CAD build for the part. Positions are in the model's coordinates, mm. A direction names the side the tool comes from. Coordinates: 2 decimals unless noted, no trailing zeros. Order: outer loops, then holes, each group sorted by start corner. A loop starts at its lowest first (then second) coordinate and runs counter-clockwise, first axis right, second up. Notation, with made-up numbers: M -38.75,32 L -22.75,32 A20 cw -22.75,38 Z; hole C 3,77.25 d9. An arc over 180 degrees is marked long. Write item = value, one per line.
Autodesk Inventor part; units mm, degrees
ref_plane "WorkPlane1" through (0, 0, 0) normal (0, 0, 1) x (1, 0, 0)
ref_plane "Work Plane2" through (0, 0, -1.3) normal (0, 0, 1) x (1, 0, 0)
ref_plane "WorkPlane2" through (0, 0, 1) normal (0, 0, 1) x (1, 0, 0)
ref_plane "WorkPlane1" through (0, 0, 0) normal (0, 0, 1) x (1, 0, 0)
ref_plane "Work Plane2" through (0, 0, -1.3) normal (0, 0, 1) x (1, 0, 0)
ref_plane "WorkPlane2" through (0, 0, 1) normal (0, 0, 1) x (1, 0, 0)
sketch "Szkic1" plane through (0, 0, 0) normal (0, 0, 1) x (1, 0, 0)
  point P0 (0, 0)
sketch "Szkic2" plane through (0, 0, 0) normal (0, 0, 1) x (1, 0, 0)
  line L0 (6.5, -14.9542) -> (5.6095, -12.8096)
  arc A0 (8.8615, -10.0274) -> (5.6095, -12.8096) centre (7.6875, -11.9468) ccw
  line L1 (8.8615, -10.0274) -> (10.3425, -10.9332)
  arc A1 (10.3425, -10.9332) -> (-10.3425, -10.9332) centre (0, 0) ccw
  line L2 (-8.8615, -10.0274) -> (-10.3425, -10.9332)
  arc A2 (-5.6095, -12.8096) -> (-8.8615, -10.0274) centre (-7.6875, -11.9468) ccw
  line L3 (-6.5, -14.9542) -> (-5.6095, -12.8096)
  arc A3 (6.5, -14.9542) -> (-6.5, -14.9542) centre (0, 0.7) ccw
  line L4 (0, 0.7) -> (-6.5, -14.9542) construction
  line L5 (0, 0.7) -> (6.5, -14.9542) construction
  dimension "d2" = 16.95
  dimension "d4" = 0
  dimension "d6" = 15.05
  dimension "d8" = 0.7
  dimension "d10" = 6.5
  dimension "d12" = 6.5
  dimension "d14" = 2.25
  dimension "d16" = 2.25
  dimension "d18" = 14.8
  dimension "d20" = 14.8
  dimension "d22" = 36
  dimension "d24" = 36
extrude "Wyciągnięcie proste1" add sketch "Szkic2" along normal blind 1.3
sketch "Szkic3" plane through (0, 0, 1.3) normal (0, 0, 1) x (1, 0, 0)
  arc A0 (-5.6095, -12.8096) -> (-8.8615, -10.0274) centre (-7.6875, -11.9468) ccw
hole "Otwór1" at (-7.6875, -11.9468, 1.3) direction (0, 0, -1) diameter 2.5 end through all
sketch "Szkic4" plane through (0, 0, 1.3) normal (0, 0, 1) x (1, 0, 0)
  arc A0 (8.8615, -10.0274) -> (5.6095, -12.8096) centre (7.6875, -11.9468) ccw
hole "Otwór2" at (7.6875, -11.9468, 1.3) direction (0, 0, -1) diameter 2.5 end through all
equation "\"d2\" = 0.5 * Diam2"
equation "\"d6\" = 0.5 * msp_dd1"
equation "\"d8\" = -0.5 * msp_dd1 + 0.5 * Diam2 - 0.222222 * ParA"
equation "\"d10\" = 2.6 * Diam5"
equation "\"d12\" = 2.6 * Diam5"
equation "\"d14\" = 0.9 * Diam5"
equation "\"d16\" = 0.9 * Diam5"
equation "\"d18\" = 1.3 * Diam5 + 0.5 * Diam2 - ParA"
equation "\"d20\" = 1.3 * Diam5 + 0.5 * Diam2 - ParA"
equation "\"d25\" = ParS"
equation "\"d29\" = Diam5"
equation "\"d36\" = Diam5"
equation "\"Diam5\" = 2.5"
equation "\"ParA\" = 5.4"
equation "\"ParS\" = 1.3"
equation "\"Diam2\" = 33.9"
equation "\"msp_dd1\" = -b + Diam2 - 0.111111 * ParA"
equation "\"msp_pom\" = 0.5 * Diam2 - b"
equation "\"TEMPLATE\" = 1.2345"
properties part number "ANSI B 27.7M - 3BMI-32" material "Stal, miękka"
(1) Slice it at C-C, the plane z = 0.4. Write the cut outline in (x, y).
Evaluation:
outline = M -10.34,-10.93 A15.05 cw long 10.34,-10.93 L 8.86,-10.03 A2.25 ccw 5.61,-12.81 L 6.5,-14.95 A16.95 ccw long -6.5,-14.95 L -5.61,-12.81 A2.25 ccw -8.86,-10.03 Z; hole C -7.69,-11.95 d2.5; hole C 7.69,-11.95 d2.5
(2) Pin check, flat tip, straight feed: pin 1 Ø10 at (x, y) = (7.5, 3) entering from +Z. Stop position of the tip, or through.
Evaluation:
pin_1 = through
(3) Slice it at D-D, the plane x = 0. Write the cut outline in (y, z).
Evaluation:
outline = M 15.05,0 L 17.65,0 L 17.65,1.3 L 15.05,1.3 Z
(4) Tool access for faces 1 (the face through (6.061, -13.897, 0.641)), 2 (the face through (-4, 15, 0)), 3 (the face through (9.592, -10.474, 0.641)): list every direction of +Z, -Z, +X, -X, +Y, -Y with a clear straight run to the whole face (end or side of a thin tool).
Evaluation:
face_1 = +Z, -Z, -Y
face_2 = -Z, +X, -X, +Y, -Y
face_3 = +Z, -Z
(5) Wall check: line 1 (X direction, y = 0.5, z = 0.5); line 2 (Y direction, x = -8.5, z = 0.3); line 3 (X direction, y = -12.5, z = 0.85). Give the ranges that are in metal, low to high. Write a range as from..to.
Evaluation:
line_1 = -16.95..-15.04, 15.04..16.95
line_2 = -13.96..-12.9, -11..-9.85, 12.42..15.36
line_3 = -10.63..-8.81, -6.57..-5.51, 5.51..6.57, 8.81..10.63
(6) Slice it at A-A, the plane y = 12. Write the cut outline in (x, z), then the cut area to 3 significant figures.
Evaluation:
outline = M -12.63,0 L -9.08,0 L -9.08,1.3 L -12.63,1.3 Z; M 9.08,0 L 12.63,0 L 12.63,1.3 L 9.08,1.3 Z
area = 9.23 mm²
(7) Slice it at B-B, the plane x = -11.5. Write the cut outline in (y, z).
Evaluation:
outline = M -11.75,0 L -9.71,0 L -9.71,1.3 L -11.75,1.3 Z; M 9.71,0 L 13.15,0 L 13.15,1.3 L 9.71,1.3 Z
(8) Pull direction X, two halves, no side cores. Call faces 4 (the face through (-0.652, 17.638, 0.641)), 5 (the face through (-4, 15, 1.3)), 6 (the face through (-9.592, -10.474, 0.641)): +X half, -X half, draft (parallel to the pull), parting line (faces both ways), or undercut.
Evaluation:
face_4 = parting line
face_5 = draft
face_6 = undercut
